```python
from build123d import *

# Parameters (mm, degrees)
F0_W   = 12.5
F0_H   = 1
F0_W_2 = 10
F0_W_3 = 15
F0_H_2 = 3


with BuildPart() as f1:
    # F0 (on Front) → F1 (revolve)
    with BuildSketch(Plane.XZ):
        with BuildLine():
            Line((0, -5.27), (12.5, -5.27))
            ThreePointArc((12.5, -5.27), (8.884681, -3.326098), (5, -2))
            ThreePointArc((5, -2), (2.702104, -0.494741), (0, 0))
            Line((0, 0), (0, -5.27))
        make_face()
        with Locations((6.25, -5.77)):
            Rectangle(F0_W, F0_H)
        Polygon((7.5, -21.27), (12.5, -6.27), (0, -6.27), (0, -21.27), align=None)
        Polygon((7.502531, -22.27), (7.5, -21.27), (0, -21.27), (0, -22.27), align=None)
        with BuildLine():
            ThreePointArc((6, -25.59), (7.822087, -24.414621), (7.502531, -22.27))
            Line((7.502531, -22.27), (0, -22.27))
            Line((0, -22.27), (0, -25.59))
            Line((0, -25.59), (6, -25.59))
        make_face()
        with BuildLine():
            ThreePointArc((6, -68.02), (3.463843, -46.805), (6, -25.59))
            Line((6, -25.59), (0, -25.59))
            Line((0, -25.59), (0, -68.02))
            Line((0, -68.02), (6, -68.02))
        make_face()
        with BuildLine():
            ThreePointArc((10, -70.02), (8.421705, -68.176591), (6, -68.02))
            Line((6, -68.02), (0, -68.02))
            Line((0, -68.02), (0, -70.02))
            Line((0, -70.02), (10, -70.02))
        make_face()
        with Locations((5, -70.52)):
            Rectangle(F0_W_2, F0_H)
        with BuildLine():
            ThreePointArc((13, -79.99), (13.690372, -74.772434), (10, -71.02))
            Line((10, -71.02), (0, -71.02))
            Line((0, -71.02), (0, -79.99))
            Line((0, -79.99), (13, -79.99))
        make_face()
        Polygon((15, -81.99), (13, -79.99), (0, -79.99), (0, -81.99), align=None)
        with Locations((7.5, -83.49)):
            Rectangle(F0_W_3, F0_H_2)
    revolve(axis=Axis((0, 0, -42.495), (0, 0, 1)))


solid = f1.part
```
Geometry check sheet. Reference: the model listing, model coordinates, mm. A direction names the side the tool comes from. Coordinates: 2 decimals unless noted, no trailing zeros. Loops run counter-clockwise (first coordinate to the right, second up) from the corner with the lowest first, then second, coordinate; pieces in that order, holes last.
Item 1: Release check for a two-part mould opening along Z. For faces 3 (the face through (-1.93, -8.71, -17)), 4 (the face through (-14.985, 0.66, -83.469)), 5 (the face through (0, 0, -84.99)) record: released by +Z, released by -Z, zero draft, split by the parting line, or undercut.
Item 2: Sectioned sample at A-A, the plane z = -73.5. Record the boundary of the cut face in (x, y).
Item 3: Access from +Z, -Z, +X, -X, +Y, -Y to the whole of each face (thin tool, end or side, straight path). Record for faces 1 (the face through (-1.7, 13, -80.1)), 2 (the face through (11.923, 3.755, -5.763)).
Item 4: Thickness scan on line 1 (Y direction, x = -2.75, z = -39); line 2 (X direction, y = -8.75, z = -12); line 3 (Y direction, x = 0, z = -46). Record the ranges inside material, lowest first.
Item 5: Go/stop test with flat-tipped pins: pin 1 Ø6 at (x, z) = (7.5, -26.5) entering from -Y; pin 2 Ø12 at (y, z) = (-10, -18.5) entering from -X; pin 3 Ø1 at (y, z) = (-7, -20) entering from -X. Record where each tip stops, or that it passes through.
Item 6: Sectioned sample at B-B, the plane z = -60.5. Record the boundary of the cut face in (x, y), then the cut area to 3 significant figures.
Check result:
1. face 3: undercut
1. face 4: zero draft
1. face 5: released by -Z
2. outline: circle Ø26.18 at (0, 0)
3. face 1: none
3. face 2: +Z
4. line 1: y = -2.63 to 2.63
4. line 2: x = -5.97 to 5.97
4. line 3: y = -3.47 to 3.47
5. pin 1: stops at y = -5.73
5. pin 2: stops at x = -8.11
5. pin 3: stops at x = -4.59
6. outline: circle Ø9.02 at (0, 0)
6. area: 64.0 mm2
